Check sheet for the modelled part. Datum: model origin and axes. Units: mm. A direction names the side the tool comes from. Give positions to 0.01 mm unless a question says otherwise; leave off trailing zeros. Write each loop counter-clockwise with the first axis right and the second up, starting at its lowest first coordinate (ties: lowest second). Pieces come first, ordered by that corner, then holes. Notation, with made-up numbers: (70.5, 49) -> (98.5, 49) arc R17 cw to (98.5, 56) -> close; hole circle Ø7 at (76.5, 20). An arc over 180 degrees is marked (long way). Use a Markdown table: item, result. Add a question column.
1. Release check for a two-part mould opening along X. For faces 4 (the flat face through (-62, 3, 18)), 5 (the flat face through (111, 3, 52)), 6 (the flat face through (95, 3, 59)), 7 (the flat face through (-95, 3, -59)) record: released by +X, released by -X, zero draft, split by the parting line, or undercut.
2. Cross-section at A-A (x = -65). Enter the section's corners in (y, z), then the cut area to 3 significant figures.
3. Gauge pin test, flat ends, axial feed: P1, Ø1, axis at y = 1, z = 52, coming from the -X side; P2, Ø1.5, axis at x = 34, y = 3.5, coming from the -Z side; P3, Ø3, axis at x = 109.5, y = 1.5, coming from the +Z side; P4, Ø1.8, axis at x = 97.6, z = 17, coming from the -Y side. Record the tip position at first contact, or that the pin passes through.
4. Set-up check for faces 1 (the flat face through (-1, 3, 52)), 2 (the flat face through (-111, 3, 52)), 3 (the flat face through (-1, 3, -52)): record each of +Z, -Z, +X, -X, +Y, -Y from which the full face is reachable in a straight line by a thin tool's end or side.
5. Cross-section at B-B (y = 1.8). Count the separate pieces of the cut face and the enclosed holes in it, then the cut area to 3 significant figures.
6. Cross-section at C-C (x = -13). Enter the section's corners in (y, z), then the cut area to 3 significant figures.
7. Scan lines: probe 1 along Z at (x, y) = (20.5, 3.4); probe 2 along X at (y, z) = (4.3, -18); probe 3 along Z at (x, y) = (-72.4, 2.4). Record each from-to range of solid material in increasing order. Write a range as [from, to].
from build123d import *

# Parameters (mm, degrees)
SKETCH_1_W          = 265
SKETCH_1_H          = 104
EXTRUDE_1_DEPTH     = 5.6
SKETCH_2_R          = 1.6
CUT_EXTRUDE_4_DEPTH = 143.448622317
SKETCH_4_R          = 1.1
SKETCH_4_W          = 10
SKETCH_4_H          = 20
CUT_EXTRUDE_6_DEPTH = 143.448622317
SKETCH_5_W          = 20
SKETCH_5_H          = 15.8
SKETCH_5_R          = 1.6
EXTRUDE_2_DEPTH     = 5.6
FILLET_1_R          = 5
FILLET_2_R          = 2


with BuildPart() as part:
    # ｽｹｯﾁ1 → ﾎﾞｽ - 押し出し1 (new body)
    with BuildSketch(Plane(origin=(0, 0, 0), x_dir=(1, 0, 0), z_dir=(0, 1, 0))):
        Rectangle(SKETCH_1_W, SKETCH_1_H)
    extrude(amount=EXTRUDE_1_DEPTH)

    # ｽｹｯﾁ2 → ｶｯﾄ - 押し出し4 (cut, through all)
    with BuildSketch(Plane(origin=(0, 0, 0), x_dir=(1, 0, 0), z_dir=(0, 1, 0))):
        with Locations(Location((20.5, 18, 0), (0, 0, 270))):
            Circle(SKETCH_2_R)
        with Locations(Location((20.5, -18, 0), (0, 0, 90))):
            Circle(SKETCH_2_R)
        with Locations(Location((-20.5, -18, 0), (0, 0, 270))):
            Circle(SKETCH_2_R)
        with Locations(Location((-20.5, 18, 0), (0, 0, 90))):
            Circle(SKETCH_2_R)
    extrude(amount=CUT_EXTRUDE_4_DEPTH, mode=Mode.SUBTRACT)

    # ｽｹｯﾁ4 → ｶｯﾄ - 押し出し6 (cut, through all)
    with BuildSketch(Plane(origin=(0, 5.6, 0), x_dir=(1, 0, 0), z_dir=(0, 1, 0))):
        with Locations(Location((97.6, 1, 0), (0, 0, 270))):
            Circle(SKETCH_4_R)
        with Locations(Location((97.6, -17, 0), (0, 0, 90))):
            Circle(SKETCH_4_R)
        with Locations(Location((52.4, 1, 0), (0, 0, 90))):
            Circle(SKETCH_4_R)
        with Locations(Location((52.4, -17, 0), (0, 0, 270))):
            Circle(SKETCH_4_R)
        with Locations(Location((-72.4, 1, 0), (0, 0, 270))):
            Circle(SKETCH_4_R)
        with Locations(Location((-72.4, -17, 0), (0, 0, 90))):
            Circle(SKETCH_4_R)
        with Locations(Location((-117.6, 1, 0), (0, 0, 90))):
            Circle(SKETCH_4_R)
        with Locations(Location((-117.6, -17, 0), (0, 0, 270))):
            Circle(SKETCH_4_R)
        with Locations((-62.4, -8)):
            Rectangle(SKETCH_4_W, SKETCH_4_H)
        with Locations((107.6, -8)):
            Rectangle(SKETCH_4_W, SKETCH_4_H)
    extrude(amount=-CUT_EXTRUDE_6_DEPTH, mode=Mode.SUBTRACT)

    # ｽｹｯﾁ5 → ﾎﾞｽ - 押し出し2 (add)
    # profile 1 of 4: a face of its own
    with BuildSketch(Plane(origin=(0, 5.6, 0), x_dir=(1, 0, 0), z_dir=(0, 1, 0))):
        with Locations((85, 59.9)):
            Rectangle(SKETCH_5_W, SKETCH_5_H)
        with Locations(Location((85, 62.8, 0), (0, 0, 270))):
            Circle(SKETCH_5_R, mode=Mode.SUBTRACT)
    # profile 2 of 4: a face of its own
    with BuildSketch(Plane(origin=(0, 5.6, 0), x_dir=(1, 0, 0), z_dir=(0, 1, 0))):
        with Locations((-85, 59.9)):
            Rectangle(SKETCH_5_W, SKETCH_5_H)
        with Locations(Location((-85, 62.8, 0), (0, 0, 90))):
            Circle(SKETCH_5_R, mode=Mode.SUBTRACT)
    # profile 3 of 4: a face of its own
    with BuildSketch(Plane(origin=(0, 5.6, 0), x_dir=(1, 0, 0), z_dir=(0, 1, 0))):
        with Locations((85, -59.9)):
            Rectangle(SKETCH_5_W, SKETCH_5_H)
        with Locations(Location((85, -62.8, 0), (0, 0, 90))):
            Circle(SKETCH_5_R, mode=Mode.SUBTRACT)
    # profile 4 of 4: a face of its own
    with BuildSketch(Plane(origin=(0, 5.6, 0), x_dir=(1, 0, 0), z_dir=(0, 1, 0))):
        with Locations((-85, -59.9)):
            Rectangle(SKETCH_5_W, SKETCH_5_H)
        with Locations(Location((-85, -62.8, 0), (0, 0, 270))):
            Circle(SKETCH_5_R, mode=Mode.SUBTRACT)
    extrude(amount=-EXTRUDE_2_DEPTH)

    # ﾌｨﾚｯﾄ1
    fillet_1_edges = [part.edges().sort_by_distance(p)[0] for p in [
        (132.5, 2.8, 52),
        (-132.5, 2.8, 52),
        (-132.5, 2.8, -52),
        (132.5, 2.8, -52),
    ]]
    fillet(fillet_1_edges, radius=FILLET_1_R)

    # ﾌｨﾚｯﾄ2
    fillet_2_edges = [part.edges().sort_by_distance(p)[0] for p in [
        (-95, 2.8, -67.8),
        (-75, 2.8, -67.8),
        (95, 2.8, 67.8),
        (75, 2.8, 67.8),
        (-75, 2.8, 67.8),
        (-95, 2.8, 67.8),
        (75, 2.8, -67.8),
        (95, 2.8, -67.8),
    ]]
    fillet(fillet_2_edges, radius=FILLET_2_R)


solid = part.part
Worked answers:
| question | item | result |
|---|---|---|
| 1 | face 4 | undercut |
| 1 | face 5 | zero draft |
| 1 | face 6 | released by +X |
| 1 | face 7 | released by -X |
| 2 | outline | (0, -52) -> (5.6, -52) -> (5.6, -2) -> (0, -2) -> close; (0, 18) -> (5.6, 18) -> (5.6, 52) -> (0, 52) -> close |
| 2 | area | 470 mm² |
| 3 | P1 | stops at x = -129.68 |
| 3 | P2 | stops at z = -52 |
| 3 | P3 | stops at z = 52 |
| 3 | P4 | passes through |
| 4 | face 1 | +Z, +Y, -Y |
| 4 | face 2 | +Z, -X, +Y, -Y |
| 4 | face 3 | -Z, +Y, -Y |
| 5 | separate pieces | 1 |
| 5 | enclosed holes | 18 |
| 5 | area | 28,300 mm² |
| 6 | outline | (0, -52) -> (5.6, -52) -> (5.6, 52) -> (0, 52) -> close |
| 6 | area | 582 mm² |
| 7 | probe 1 | z = [-52, -19.6], [-16.4, 16.4], [19.6, 52] |
| 7 | probe 2 | x = [-132.5, -22.1], [-18.9, 18.9], [22.1, 132.5] |
| 7 | probe 3 | z = [-52, -2.1], [0.1, 15.9], [18.1, 52] |
